Autodesk Inventor part; units mm, degrees
ref_plane "YZ Plane" through (0, 0, 0) normal (1, 0, 0) x (0, 1, 0)
ref_plane "XZ Plane" through (0, 0, 0) normal (0, 1, 0) x (-1, 0, 0)
ref_plane "XY Plane" through (0, 0, 0) normal (0, 0, 1) x (1, 0, 0)
sketch "Эскиз1" plane through (0, 0, 0) normal (0, 1, 0) x (-1, 0, 0)
  line L0 (-21.15, 21.15) -> (21.15, 21.15)
  line L1 (21.15, 21.15) -> (21.15, -21.15)
  line L2 (21.15, -21.15) -> (-21.15, -21.15)
  line L3 (-21.15, -21.15) -> (-21.15, 21.15)
  line L4 (-21.15, 21.15) -> (21.15, -21.15) construction
  line L5 (21.15, 21.15) -> (-21.15, -21.15) construction
  line L6 (-23.15, 23.15) -> (23.15, 23.15)
  line L7 (23.15, 23.15) -> (23.15, -23.15)
  line L8 (23.15, -23.15) -> (-23.15, -23.15)
  line L9 (-23.15, -23.15) -> (-23.15, 23.15)
  line L10 (-23.15, 23.15) -> (23.15, -23.15) construction
  line L11 (23.15, 23.15) -> (-23.15, -23.15) construction
  point P0 (0, 0)
  dimension "d0" = 42.3
  dimension "d1" = 42.3
  dimension "d2" = 46.3
  dimension "d3" = 46.3
extrude "Выдавливание1" add sketch "Эскиз1" along normal blind 48
sketch "Эскиз2" plane through (23.15, 0, 23.15) normal (1, 0, 0) x (0, 0, -1)
  line L0 (23.15, 9.5) -> (36.05, 9.5)
  line L1 (36.05, 9.5) -> (10.25, 9.5)
  line L2 (10.25, 9.5) -> (10.25, 0)
  line L3 (44.3, 0) -> (2, 0)
  line L4 (36.05, 9.5) -> (36.05, 0)
  point P0 (23.15, 0)
  dimension "d6" = 9.5
  dimension "d7" = 12.9
  dimension "d8" = 25.8
extrude "Выдавливание2" cut sketch "Эскиз2" against normal blind 2
sketch "Эскиз3" plane through (0, 48, 0) normal (0, 1, 0) x (1, 0, 0)
  line L0 (-23.15, 23.15) -> (-23.15, -23.15)
  line L1 (23.15, -23.15) -> (-23.15, -23.15)
  line L2 (-23.15, -23.15) -> (-23.15, 23.15)
  line L3 (-23.15, 23.15) -> (23.15, 23.15)
  line L4 (23.15, 23.15) -> (23.15, -23.15)
  line L5 (23.15, -23.15) -> (-23.15, 23.15) construction
  line L6 (-23.15, -23.15) -> (23.15, 23.15) construction
  point P0 (0, 0)
extrude "Выдавливание3" add sketch "Эскиз3" along normal blind 1.5
sketch "Эскиз4" plane through (0, 49.5, 0) normal (0, 1, 0) x (1, 0, 0)
  circle A0 centre (0, 0) radius 11.25
  line L0 (15.5, 15.5) -> (-15.5, 15.5)
  line L1 (-15.5, 15.5) -> (-15.5, -15.5)
  line L2 (-15.5, -15.5) -> (15.5, -15.5)
  line L3 (15.5, -15.5) -> (15.5, 15.5)
  line L4 (15.5, 15.5) -> (-15.5, -15.5) construction
  line L5 (-15.5, 15.5) -> (15.5, -15.5) construction
  circle A1 centre (-15.5, -15.5) radius 2
  circle A2 centre (-15.5, 15.5) radius 2
  circle A3 centre (15.5, 15.5) radius 2
  circle A4 centre (15.5, -15.5) radius 2
  dimension "d13" = 22.5
  dimension "d14" = 31
  dimension "d15" = 31
  dimension "d16" = 4
  dimension "d17" = 4
  dimension "d18" = 4
  dimension "d19" = 4
extrude "Выдавливание4" cut sketch "Эскиз4" against normal blind 1.5 contours A0 | A2 L1 L0 | L0 L1 A2 | A3 L3 L0 | L0 L3 A3 | A1 L2 L1 | L1 L2 A1 | A4 L2 L3 | L3 L2 A4
properties part number "Корпус для двигателя"
Geometry check sheet. Reference: the model listing, model coordinates, mm. A direction names the side the tool comes from. Coordinates: 2 decimals unless noted, no trailing zeros. Order: outer loops, then holes, each group sorted by start corner. A loop starts at its lowest first (then second) coordinate and runs counter-clockwise, first axis right, second up. Notation, with made-up numbers: (79.5, 47) - (100.5, 47) arc R31 ccw to (100.5, 80) - close; hole circle Ø3 at (59.25, 23). An arc over 180 degrees is marked (long way). One line per item, written item: value.
(1) Depth check by flat-ended pin: pin 1 Ø5 at (x, z) = (15.5, -15.5) entering from -Y; pin 2 Ø1 at (x, z) = (22.5, 5.5) entering from -Y. Enter the tip coordinate at first touch or a pass-through.
Data:
pin 1: stops at y = 48
pin 2: stops at y = 9.5
(2) Sectioned sample at D-D (z = 15.5). Enter the section's corners in (x, y).
Data:
outline: (-23.15, 0) - (-21.15, 0) - (-21.15, 48) - (-17.5, 48) - (-17.5, 49.5) - (-23.15, 49.5) - close; (-13.5, 48) - (13.5, 48) - (13.5, 49.5) - (-13.5, 49.5) - close; (17.5, 48) - (21.15, 48) - (21.15, 0) - (23.15, 0) - (23.15, 49.5) - (17.5, 49.5) - close
(3) Release check for a two-part mould opening along Z. For faces 1 (the face through (-22, 0, 0)), 2 (the face through (0, 24, -23.15)), 3 (the face through (21.15, 24, 0)) record: +Z half, -Z half, draft (parallel to the pull), parting line (faces both ways), or undercut.
Data:
face 1: draft
face 2: -Z half
face 3: undercut
(4) Thickness scan on probe 1 along X at (y, z) = (48.35, -15.5); probe 2 along Z at (x, y) = (-10, 2.5). Record the ranges inside material, lowest first. Write a range as from..to.
Data:
probe 1: x = -23.15..-17.5, -13.5..13.5, 17.5..23.15
probe 2: z = -23.15..-21.15, 21.15..23.15
(5) Access from +Z, -Z, +X, -X, +Y, -Y to the whole of each face (thin tool, end or side, straight path). Record for faces 4 (the face through (0, 24, -21.15)), 5 (the face through (22, 5, 12.9)), 6 (the face through (-5, 49.5, -11)).
Data:
face 4: -Y
face 5: +X, -Y
face 6: +Z, -Z, +X, -X, +Y
(6) Sectioned sample at C-C (y = 36). Enter the section's corners in (x, z), and give its area (3 significant figures).
Data:
outline: (-23.15, -23.15) - (23.15, -23.15) - (23.15, 23.15) - (-23.15, 23.15) - close; hole (-21.15, -21.15) - (21.15, -21.15) - (21.15, 21.15) - (-21.15, 21.15) - close
area: 354 mm^2
(7) Sectioned sample at A-A (z = 0). Enter the section's corners in (x, y).
Data:
outline: (-23.15, 0) - (-21.15, 0) - (-21.15, 48) - (-11.25, 48) - (-11.25, 49.5) - (-23.15, 49.5) - close; (11.25, 48) - (21.15, 48) - (21.15, 9.5) - (23.15, 9.5) - (23.15, 49.5) - (11.25, 49.5) - close
(8) Sectioned sample at B-B (x = 15.5). Enter the section's corners in (y, z).
Data:
outline: (0, -23.15) - (49.5, -23.15) - (49.5, -17.5) - (48, -17.5) - (48, -21.15) - (0, -21.15) - close; (0, 21.15) - (48, 21.15) - (48, 17.5) - (49.5, 17.5) - (49.5, 23.15) - (0, 23.15) - close; (48, -13.5) - (49.5, -13.5) - (49.5, 13.5) - (48, 13.5) - close
